from build123d import *

# Parameters (mm, degrees)
SKETCH1_W           = 39
SKETCH1_H           = 19
SKETCH1_W_2         = 37
SKETCH1_H_2         = 17
BOSS_EXTRUDE1_DEPTH = 7
BOSS_EXTRUDE2_DEPTH = 1
BOSS_EXTRUDE3_START = 8
BOSS_EXTRUDE3_DEPTH = 8
SKETCH4_W           = 8
SKETCH4_H           = 7
CUT_EXTRUDE1_DEPTH  = 8


with BuildPart() as part:
    # Sketch1 → Boss-Extrude1 (new body)
    with BuildSketch(Plane(origin=(0, 0, 0), x_dir=(1, 0, 0), z_dir=(0, 1, 0))):
        with Locations((32.618409138, 12.656662155)):
            Rectangle(SKETCH1_W, SKETCH1_H)
        with Locations((32.618409138, 12.656662155)):
            Rectangle(SKETCH1_W_2, SKETCH1_H_2, mode=Mode.SUBTRACT)
    extrude(amount=BOSS_EXTRUDE1_DEPTH)

    # Sketch2 → Boss-Extrude2 (add)
    with BuildSketch(Plane.XZ):
        with BuildLine():
            Line((13.118409138, -3.156662155), (30.868409138, -3.156662155))
            ThreePointArc((30.868409138, -3.156662155), (32.618409138, -1.406662155), (34.368409138, -3.156662155))
            Line((34.368409138, -3.156662155), (52.118409138, -3.156662155))
            Line((52.118409138, -3.156662155), (52.118409138, -22.156662155))
            Line((52.118409138, -22.156662155), (34.368409138, -22.156662155))
            ThreePointArc((34.368409138, -22.156662155), (32.618409138, -23.906662155), (30.868409138, -22.156662155))
            Line((30.868409138, -22.156662155), (13.118409138, -22.156662155))
            Line((13.118409138, -22.156662155), (13.118409138, -3.156662155))
        make_face()
    extrude(amount=BOSS_EXTRUDE2_DEPTH)

    # Sketch3 → Boss-Extrude3 (add)
    with BuildSketch(Plane(origin=(0, 0, 0), x_dir=(1, 0, 0), z_dir=(0, 1, 0)).offset(BOSS_EXTRUDE3_START)):
        with BuildLine():
            Line((30.868409138, 22.156662155), (34.368409138, 22.156662155))
            ThreePointArc((34.368409138, 22.156662155), (32.618409138, 23.906662155), (30.868409138, 22.156662155))
        make_face()
        with BuildLine():
            Line((30.868409138, 3.156662155), (34.368409138, 3.156662155))
            ThreePointArc((34.368409138, 3.156662155), (32.618409138, 1.406662155), (30.868409138, 3.156662155))
        make_face()
    extrude(amount=-BOSS_EXTRUDE3_DEPTH)

    # Sketch4 → Cut-Extrude1 (cut)
    with BuildSketch(Plane(origin=(52.118409138, 0, 0), x_dir=(0, 0, -1), z_dir=(1, 0, 0))):
        with Locations((12.656662155, 3.5)):
            Rectangle(SKETCH4_W, SKETCH4_H)
    extrude(amount=-CUT_EXTRUDE1_DEPTH, mode=Mode.SUBTRACT)


solid = part.part
Work out the finished part from the listing and answer in its coordinate system (mm). A direction names the side the tool comes from. Give positions to 0.01 mm unless a question says otherwise; leave off trailing zeros. Loops run counter-clockwise (first coordinate to the right, second up) from the corner with the lowest first, then second, coordinate; pieces in that order, holes last. Notation, with made-up numbers: M 33.25,7.25 L 90.25,7.25 A11 cw 90.25,25.25 Z; hole C 45,15.25 d8. An arc over 180 degrees is marked long. Use CSV: the item, a comma, the result in double quotes.
1) Find section C-C on y = 2. Write down the section's boundary in (x, z), plus the area to 3 significant figures.
Answer:
outline,"M 13.12,-22.16 L 30.87,-22.16 A1.75 ccw 34.37,-22.16 L 52.12,-22.16 L 52.12,-16.66 L 51.12,-16.66 L 51.12,-21.16 L 14.12,-21.16 L 14.12,-4.16 L 51.12,-4.16 L 51.12,-8.66 L 52.12,-8.66 L 52.12,-3.16 L 34.37,-3.16 A1.75 ccw 30.87,-3.16 L 13.12,-3.16 Z"
area,"114 mm^2"
2) Which of the six approach directions +Z, -Z, +X, -X, +Y, -Y give full straight-line access (tool end or side, diameter ignored) to faces 5 (the flat face through (51.118, 3, -6)), 6 (the flat face through (51.6, 3.5, -16.657)), 7 (the flat face through (32.6, 7.5, -22.157)), 8 (the flat face through (43, 3, -3.157)), 9 (the flat face through (13.118, 3, -13))?
Answer:
face 5,"+Y"
face 6,"+X, +Y"
face 7,"+X, -X, +Y"
face 8,"+Z, +X, +Y, -Y"
face 9,"+Z, -Z, -X, +Y, -Y"
3) Find section A-A on z = -7.5. Write down the section's boundary in (x, y).
Answer:
outline,"M 13.12,-1 L 52.12,-1 L 52.12,7 L 51.12,7 L 51.12,0 L 14.12,0 L 14.12,7 L 13.12,7 Z"
4) Consider L1, parallel to X at y = 6, z = -20.5; L2, parallel to Z at x = 21.5, y = 1.5; L3, parallel to Y at x = 26, z = -18.25. Determine where each line is inside the solid, lowest interval first.
Answer:
L1,"13.12 to 14.12, 51.12 to 52.12"
L2,"-22.16 to -21.16, -4.16 to -3.16"
L3,"-1 to 0"
5) Given P1, Ø9.5, axis at x = 39.5, z = -15.5, coming from the +Y side; P2, Ø3.5, axis at x = 36.5, y = 4, coming from the -Z side; P3, Ø0.8, axis at x = 32, y = 7.5, coming from the -Z side, each flat-ended and moving along its own axis, determine where each tip first touches the part or whether it passes through.
Answer:
P1,"y = 0"
P2,"z = -22.16"
P3,"z = -23.89"
6) Determine the mould class of faces 1 (the flat face through (22, 3, -3.157)), 2 (the flat face through (43, 3, -22.157)), 3 (the flat face through (33, -1, -12)), 4 (the flat face through (33, 0, -13)) for opening direction Z: released by +Z, released by -Z, zero draft, split by the parting line, or undercut.
Answer:
face 1,"released by +Z"
face 2,"released by -Z"
face 3,"zero draft"
face 4,"undercut"
7) Find section D-D on z = -21.75. Write down the section's boundary in (x, y).
Answer:
outline,"M 13.12,-1 L 52.12,-1 L 52.12,7 L 13.12,7 Z"
8) Find section B-B on x = 49. Write down the section's boundary in (y, z), plus the area to 3 significant figures.
Answer:
outline,"M -1,-22.16 L 7,-22.16 L 7,-21.16 L 0,-21.16 L 0,-4.16 L 7,-4.16 L 7,-3.16 L -1,-3.16 Z"
area,"33.0 mm^2"
